from build123d import *

# Parameters (mm, degrees)
EXTRUDE_1_DEPTH      = 10
EXTRUDE_1_DEPTH_BACK = 10
SKETCH_1_W           = 1200
SKETCH_1_H           = 20
SKETCH_2_W           = 17.726991081
SKETCH_2_H           = 17.586856765
CUT_EXTRUDE_1_DEPTH  = 1201.208315252
CUT_EXTRUDE_2_REACH  = 1202.333
CUT_EXTRUDE_3_REACH  = 1202.333
CUT_EXTRUDE_4_REACH  = 1202.208
SKETCH_5_R           = 6


with BuildPart() as part:
    # Sketch 1 → Extrude 1 (new, two sides: drawn at the far end of the back side and taken through both)
    with BuildSketch(Plane.XY.offset(-EXTRUDE_1_DEPTH_BACK)):
        with Locations((600, 10)):
            Rectangle(SKETCH_1_W, SKETCH_1_H)
    extrude(amount=EXTRUDE_1_DEPTH + EXTRUDE_1_DEPTH_BACK)

    # Sketch 2 → Cut-Extrude 1 (cut, through all)
    with BuildSketch(Plane(origin=(1200, 0, 0), x_dir=(0, 0, -1), z_dir=(1, 0, 0))):
        with Locations((0.363495541, 9.706571617)):
            Rectangle(SKETCH_2_W, SKETCH_2_H)
    extrude(amount=-CUT_EXTRUDE_1_DEPTH, mode=Mode.SUBTRACT)

    # Sketch 3 → Cut-Extrude 2 (cut, up to next)
    with BuildSketch(Plane.XY.offset(10), mode=Mode.PRIVATE) as cut_extrude_2_sk1:
        with BuildLine():
            Line((91, 12.5), (109, 12.5))
            ThreePointArc((109, 12.5), (112.5, 9), (109, 5.5))
            Line((109, 5.5), (91, 5.5))
            ThreePointArc((91, 5.5), (87.5, 9), (91, 12.5))
        make_face()
    cut_extrude_2_tool1 = extrude(cut_extrude_2_sk1.sketch, amount=-CUT_EXTRUDE_2_REACH, mode=Mode.PRIVATE) & part.part
    add(cut_extrude_2_tool1.solids().sort_by_distance((100, 9, 10))[0], mode=Mode.SUBTRACT)

    # Sketch 4 → Cut-Extrude 3 (cut, up to next)
    with BuildSketch(Plane.XY.offset(10), mode=Mode.PRIVATE) as cut_extrude_3_sk1:
        with BuildLine():
            Line((1091, 12.5), (1109, 12.5))
            ThreePointArc((1109, 12.5), (1112.5, 9), (1109, 5.5))
            Line((1109, 5.5), (1091, 5.5))
            ThreePointArc((1091, 5.5), (1087.5, 9), (1091, 12.5))
        make_face()
    cut_extrude_3_tool1 = extrude(cut_extrude_3_sk1.sketch, amount=-CUT_EXTRUDE_3_REACH, mode=Mode.PRIVATE) & part.part
    add(cut_extrude_3_tool1.solids().sort_by_distance((1100, 9, 10))[0], mode=Mode.SUBTRACT)

    # Sketch 5 → Cut-Extrude 4 (cut, up to next)
    with BuildSketch(Plane.XZ, mode=Mode.PRIVATE) as cut_extrude_4_sk1:
        with Locations(Location((600, 0, 0), (0, 0, 270))):
            Circle(SKETCH_5_R)
    cut_extrude_4_tool1 = extrude(cut_extrude_4_sk1.sketch, amount=-CUT_EXTRUDE_4_REACH, mode=Mode.PRIVATE) & part.part
    add(cut_extrude_4_tool1.solids().sort_by_distance((600, 0, 0))[0], mode=Mode.SUBTRACT)


solid = part.part
Read the model definition and answer for the solid it produces. Units are mm, in the model's axes. Round coordinates to 2 decimals unless told otherwise and drop trailing zeros. Write each loop counter-clockwise with the first axis right and the second up, starting at its lowest first coordinate (ties: lowest second). Pieces come first, ordered by that corner, then holes. Notation, with made-up numbers: M 10.5,-12 L 62.5,-12 A34 cw 62.5,20 Z; hole C -11,69 d5. An arc over 180 degrees is marked long. Use a Markdown table: item, result.
1) Straight lines are drawn through the part: line 1 along Z through (x, y) = (601.5, 5.5); line 2 along Y through (x, z) = (76.5, -9); line 3 along X through (y, z) = (0.55, 0). For each, find the intervals that lie inside material, in ascending order. Write a range as [from, to].
Answers follow:
| item | result |
|---|---|
| line 1 | z = [-10, -9.23], [8.5, 10] |
| line 2 | y = [0, 0.91], [18.5, 20] |
| line 3 | x = [0, 594], [606, 1200] |
2) The part is cut by section A-A (z = 0). Write down the section's boundary in (x, y).
Answers follow:
| item | result |
|---|---|
| outline | M 0,0 L 594,0 L 594,0.91 L 0,0.91 Z; M 0,18.5 L 1200,18.5 L 1200,20 L 0,20 Z; M 606,0 L 1200,0 L 1200,0.91 L 606,0.91 Z |
3) Flat-ended cylindrical pins translate along their axes: pin 1 (11 mm diameter, centred on x = 600, z = 0, fed in from -Y); pin 2 (2 mm diameter, centred on y = 10, z = -6.5, fed in from +X). Find the tip coordinate at first contact, or state that the pin passes through.
Answers follow:
| item | result |
|---|---|
| pin 1 | stops at y = 18.5 |
| pin 2 | passes through |
4) The part is cut by section C-C (x = 960.5). Write down the section's boundary in (y, z), plus the area to 3 significant figures.
Answers follow:
| item | result |
|---|---|
| outline | M 0,-10 L 20,-10 L 20,10 L 0,10 Z; hole M 0.91,-9.23 L 18.5,-9.23 L 18.5,8.5 L 0.91,8.5 Z |
| area | 88.2 mm2 |
5) The part is cut by section B-B (y = 9). Write down the section's boundary in (x, z), plus the area to 3 significant figures.
Answers follow:
| item | result |
|---|---|
| outline | M 0,-10 L 1200,-10 L 1200,-9.23 L 0,-9.23 Z; M 0,8.5 L 87.5,8.5 L 87.5,10 L 0,10 Z; M 112.5,8.5 L 1087.5,8.5 L 1087.5,10 L 112.5,10 Z; M 1112.5,8.5 L 1200,8.5 L 1200,10 L 1112.5,10 Z |
| area | 2,650 mm2 |
